from build123d import *

# Parameters (mm, degrees)
BOSS_EXTRUDE1_DEPTH = 50
CUT_EXTRUDE1_REACH  = 101.499
SKETCH3_R           = 11
SKETCH3_R_2         = 1.5


with BuildPart() as part:
    # Sketch1 → Boss-Extrude1 (new body)
    with BuildSketch(Plane(origin=(0, 0, 0), x_dir=(0, 0, -1), z_dir=(1, 0, 0))):
        Polygon((0, 0), (0, 50), (5, 50), (5, 5), (70, 5), (70, 0), align=None)
    extrude(amount=BOSS_EXTRUDE1_DEPTH)

    # Sketch3 → Cut-Extrude1 (cut, up to next)
    with BuildSketch(Plane.XY, mode=Mode.PRIVATE) as cut_extrude1_sk1:
        with Locations((25, 25)):
            Circle(SKETCH3_R)
    cut_extrude1_tool1 = extrude(cut_extrude1_sk1.sketch, amount=-CUT_EXTRUDE1_REACH, mode=Mode.PRIVATE) & part.part
    # Sketch3 → Cut-Extrude1 (cut, up to next)
    with BuildSketch(Plane.XY, mode=Mode.PRIVATE) as cut_extrude1_sk2:
        with Locations((40.5, 40.5)):
            Circle(SKETCH3_R_2)
    cut_extrude1_tool2 = extrude(cut_extrude1_sk2.sketch, amount=-CUT_EXTRUDE1_REACH, mode=Mode.PRIVATE) & part.part
    # Sketch3 → Cut-Extrude1 (cut, up to next)
    with BuildSketch(Plane.XY, mode=Mode.PRIVATE) as cut_extrude1_sk3:
        with Locations((9.5, 40.5)):
            Circle(SKETCH3_R_2)
    cut_extrude1_tool3 = extrude(cut_extrude1_sk3.sketch, amount=-CUT_EXTRUDE1_REACH, mode=Mode.PRIVATE) & part.part
    # Sketch3 → Cut-Extrude1 (cut, up to next)
    with BuildSketch(Plane.XY, mode=Mode.PRIVATE) as cut_extrude1_sk4:
        with Locations((9.5, 9.5)):
            Circle(SKETCH3_R_2)
    cut_extrude1_tool4 = extrude(cut_extrude1_sk4.sketch, amount=-CUT_EXTRUDE1_REACH, mode=Mode.PRIVATE) & part.part
    # Sketch3 → Cut-Extrude1 (cut, up to next)
    with BuildSketch(Plane.XY, mode=Mode.PRIVATE) as cut_extrude1_sk5:
        with Locations((40.5, 9.5)):
            Circle(SKETCH3_R_2)
    cut_extrude1_tool5 = extrude(cut_extrude1_sk5.sketch, amount=-CUT_EXTRUDE1_REACH, mode=Mode.PRIVATE) & part.part
    add(cut_extrude1_tool1.solids().sort_by_distance((25, 25, 0))[0], mode=Mode.SUBTRACT)
    add(cut_extrude1_tool2.solids().sort_by_distance((40.5, 40.5, 0))[0], mode=Mode.SUBTRACT)
    add(cut_extrude1_tool3.solids().sort_by_distance((9.5, 40.5, 0))[0], mode=Mode.SUBTRACT)
    add(cut_extrude1_tool4.solids().sort_by_distance((9.5, 9.5, 0))[0], mode=Mode.SUBTRACT)
    add(cut_extrude1_tool5.solids().sort_by_distance((40.5, 9.5, 0))[0], mode=Mode.SUBTRACT)


solid = part.part
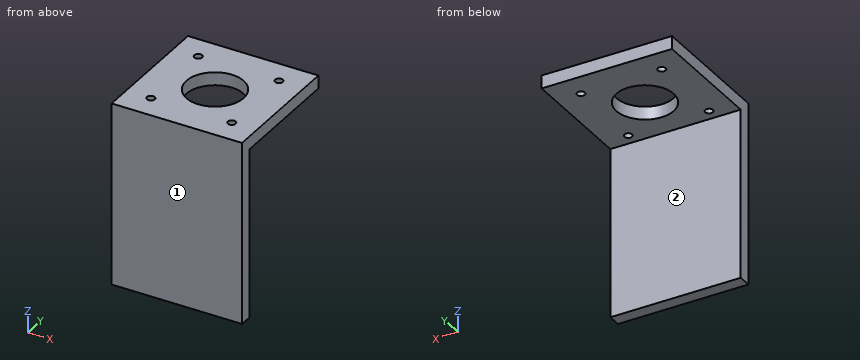
Read the model definition and answer for the solid it produces. Units are mm, in the model's axes. Face numbers are marked on the shaded views. A direction names the side the tool comes from. Give positions to 0.01 mm unless a question says otherwise; leave off trailing zeros. Write each loop counter-clockwise with the first axis right and the second up, starting at its lowest first coordinate (ties: lowest second). Pieces come first, ordered by that corner, then holes. Notation, with made-up numbers: (64, 52.5) - (79, 52.5) arc R5 cw to (79, 56.5) - close; hole circle Ø1 at (-4, -31). An arc over 180 degrees is marked (long way). Use CSV: the item, a comma, the result in double quotes. Start each with the question number.
(1) Find section D-D (z = -51). Give the vertices of the cut face in (x, y), plus the area to 3 significant figures.
(2) Find section A-A (y = 25). Give the vertices of the cut face in (x, z), plus the area to 3 significant figures.
(3) Given P1, Ø10, axis at x = 44, z = -51.5, coming from the -Y side; P2, Ø12, axis at x = 17, y = 44, coming from the -Z side; P3, Ø25, axis at x = 29, z = -41.5, coming from the +Y side, each flat-ended and moving along its own axis, determine where each tip first touches the part or whether it passes through.
(4) Find section B-B (x = 9.5). Give the vertices of the cut face in (y, z), plus the area to 3 significant figures.
(5) Find section C-C (x = 25). Give the vertices of the cut face in (y, z), plus the area to 3 significant figures.
(6) Consider line 1 along Y through (x, z) = (9.5, -1.75); line 2 along Y through (x, z) = (9, -1). Determine where each line is inside the solid, lowest interval first.
(7) For the marked faces 1 and 2, determine the directions among +Z, -Z, +X, -X, +Y, -Y from which every point of the face is accessible in a straight line to the end or side of a thin tool.
Findings below:
1,outline,"(0, 0) - (50, 0) - (50, 5) - (0, 5) - close"
1,area,"250 mm2"
2,outline,"(0, -5) - (14, -5) - (14, 0) - (0, 0) - close; (36, -5) - (50, -5) - (50, 0) - (36, 0) - close"
2,area,"140 mm2"
3,P1,"y = 0"
3,P2,"z = -5"
3,P3,"y = 5"
4,outline,"(0, -70) - (5, -70) - (5, -5) - (8, -5) - (8, 0) - (0, 0) - close; (11, -5) - (39, -5) - (39, 0) - (11, 0) - close; (42, -5) - (50, -5) - (50, 0) - (42, 0) - close"
4,area,"545 mm2"
5,outline,"(0, -70) - (5, -70) - (5, -5) - (14, -5) - (14, 0) - (0, 0) - close; (36, -5) - (50, -5) - (50, 0) - (36, 0) - close"
5,area,"465 mm2"
6,line 1,"0 to 8, 11 to 39, 42 to 50"
6,line 2,"0 to 8.09, 10.91 to 39.09, 41.91 to 50"
7,face 1,"+Z, -Z, +X, -X, -Y"
7,face 2,"-Z, +X, -X, +Y"
